Check sheet for the modelled part. Datum: model origin and axes. Units: mm. A direction names the side the tool comes from. Coordinates: 2 decimals unless noted, no trailing zeros. Order: outer loops, then holes, each group sorted by start corner. A loop starts at its lowest first (then second) coordinate and runs counter-clockwise, first axis right, second up.
1. Gauge pin test, flat ends, axial feed: pin 1 Ø12 at (x, y) = (13, -11) entering from -Z; pin 2 Ø2 at (x, y) = (4, -2.5) entering from +Z; pin 3 Ø8 at (x, y) = (24.5, -10.5) entering from +Z; pin 4 Ø5 at (x, z) = (12.5, 9) entering from -Y. Record the tip position at first contact, or that the pin passes through.
2. Draft check along Z on faces 3 (the flat face through (19, 0, 13)), 4 (the flat face through (18.42, -6.8, 17.43)), 5 (the flat face through (19, -7, 0)). Enter one of: released by +Z, released by -Z, zero draft, split by the parting line, or undercut.
3. Cross-section at C-C (z = 12). Enter the section's corners in (x, y), then the cut area to 3 significant figures.
4. Set-up check for faces 1 (the flat face through (18, -7.112, 9)), 2 (the flat face through (18.783, -6.875, 18.515)): record each of +Z, -Z, +X, -X, +Y, -Y from which the full face is reachable in a straight line by a thin tool's end or side.
5. Cross-section at D-D (y = -10). Enter the section's corners in (x, z).
6. Cross-section at A-A (y = -13.75). Enter the section's corners in (x, z).
7. Thickness scan on line 1 (X direction, y = -8.5, z = 9.5); line 2 (Y direction, x = 16, z = 7); line 3 (Y direction, x = 16, z = 19.25). Record the ranges inside material, lowest first.
8. Cross-section at B-B (x = 21.5). Enter the section's corners in (y, z), then the cut area to 3 significant figures.
```python
from build123d import *

# Parameters (mm, degrees)
F1_DEPTH = 38.1
F2_W     = 25.3906301223
F2_H     = 25.4694648265
F3_DEPTH = 12.7
F4_W     = 25.981107261
F4_H     = 16.8286710978
F5_DEPTH = 7.112


with BuildPart() as f1:
    # F0 (on Right) → F1 (new body)
    with BuildSketch(Plane.YZ):
        Polygon((-25.3906268626, 0), (0, 0), (0, 25.3906268626), align=None)
    extrude(amount=F1_DEPTH)

    # F2 (on face) → F3 (cut, symmetric)
    with BuildSketch(Plane(origin=(0, -12.6953134313, 12.6953134313), x_dir=(1, 0, 0), z_dir=(0, -0.7071067812, 0.7071067812))):
        with Locations((18.6001111288, -5.2191520199)):
            Rectangle(F2_W, F2_H)
    extrude(amount=F3_DEPTH, both=True, mode=Mode.SUBTRACT)

    # F4 (on Front) → F5 (join)
    with BuildSketch(Plane.XZ):
        with Locations((18.8953496981, 8.4143355489)):
            Rectangle(F4_W, F4_H)
    extrude(amount=F5_DEPTH)


solid = f1.part
```
Data:
1. pin 1: stops at z = 0
1. pin 2: stops at z = 23.89
1. pin 3: stops at z = 18.89
1. pin 4: stops at y = -7.11
2. face 3: zero draft
2. face 4: undercut
2. face 5: released by -Z
3. outline: (0, -13.39) - (5.9, -13.39) - (5.9, -7.11) - (31.3, -7.11) - (31.3, -13.39) - (38.1, -13.39) - (38.1, 0) - (0, 0) - close
3. area: 351 mm2
4. face 1: -Y
4. face 2: +Z, +X, -X, -Y
5. outline: (0, 0) - (5.9, 0) - (5.9, 15.39) - (0, 15.39) - close; (31.3, 0) - (38.1, 0) - (38.1, 15.39) - (31.3, 15.39) - close
6. outline: (0, 0) - (5.9, 0) - (5.9, 11.64) - (0, 11.64) - close; (31.3, 0) - (38.1, 0) - (38.1, 11.64) - (31.3, 11.64) - close
7. line 1: x = 0 to 5.9, 31.3 to 38.1
7. line 2: y = -7.11 to 0
7. line 3: y = -6.14 to 0
8. outline: (-7.43, 0) - (0, 0) - (0, 25.39) - (-7.38, 18.01) - (-6.2, 16.83) - (-7.11, 16.83) - (-7.11, 0.32) - close
8. area: 155 mm2
